from build123d import *

# Parameters (mm, degrees)
SKIZZE1_W                       = 40
SKIZZE1_H                       = 15
SKIZZE1_R                       = 1.75
AUFSATZ_LINEAR_AUSTRAGEN1_DEPTH = 1
FASE1_SIZE                      = 2


with BuildPart() as part:
    # Skizze1 → Aufsatz-Linear austragen1 (new body)
    with BuildSketch(Plane.XY):
        Rectangle(SKIZZE1_W, SKIZZE1_H)
        with Locations((-15, 0)):
            Circle(SKIZZE1_R, mode=Mode.SUBTRACT)
        with Locations((15, 0)):
            Circle(SKIZZE1_R, mode=Mode.SUBTRACT)
    extrude(amount=AUFSATZ_LINEAR_AUSTRAGEN1_DEPTH)

    # Fase1
    fase1_edges = [part.edges().sort_by_distance(p)[0] for p in [
        (-20, 7.5, 0.5),
        (20, 7.5, 0.5),
        (20, -7.5, 0.5),
        (-20, -7.5, 0.5),
    ]]
    chamfer(fase1_edges, length=FASE1_SIZE)


solid = part.part
CAD build for the part. Positions are in the model's coordinates, mm. Round coordinates to 2 decimals unless told otherwise and drop trailing zeros. Order: outer loops, then holes, each group sorted by start corner. A loop starts at its lowest first (then second) coordinate and runs counter-clockwise, first axis right, second up. Notation, with made-up numbers: (6, 38) - (32, 38) arc R24 cw to (32, 70) - close; hole circle Ø10 at (44.25, 38). An arc over 180 degrees is marked (long way). Return JSON: item names as keys, results as strings.
(1) Cut at C-C (y = 0). Give the cut face in (x, z), then the cut area to 3 significant figures.
Answer key:
{"outline": "(-20, 0) - (-16.75, 0) - (-16.75, 1) - (-20, 1) - close; (-13.25, 0) - (13.25, 0) - (13.25, 1) - (-13.25, 1) - close; (16.75, 0) - (20, 0) - (20, 1) - (16.75, 1) - close", "area": "33.0 mm^2"}
(2) Wall check: probe 1 along Y at (x, z) = (-15, 0.5); probe 2 along Y at (x, z) = (-13.5, 0.9); probe 3 along X at (y, z) = (5.75, 0.45). Give the ranges that are in metal, low to high. Write a range as from..to.
Answer key:
{"probe 1": "y = -7.5..-1.75, 1.75..7.5", "probe 2": "y = -7.5..-0.9, 0.9..7.5", "probe 3": "x = -19.75..19.75"}
(3) Pin check, flat tip, straight feed: pin 1 Ø4.5 at (x, y) = (-15, 0) entering from -Z. Stop position of the tip, or through.
Answer key:
{"pin 1": "stops at z = 0"}
(4) Cut at B-B (z = 0.25). Give the cut face in (x, y).
Answer key:
{"outline": "(-20, -5.5) - (-18, -7.5) - (18, -7.5) - (20, -5.5) - (20, 5.5) - (18, 7.5) - (-18, 7.5) - (-20, 5.5) - close; hole circle Ø3.5 at (-15, 0); hole circle Ø3.5 at (15, 0)"}
(5) Pull direction X, two halves, no side cores. Call faces 1 (the face through (-20, -0.1, 0.5)), 2 (the face through (19, -6.5, 0.5)), 3 (the face through (-13.331, 0.526, 0.493)): +X half, -X half, draft (parallel to the pull), parting line (faces both ways), or undercut.
Answer key:
{"face 1": "-X half", "face 2": "+X half", "face 3": "undercut"}
(6) Cut at A-A (x = -15). Give the cut face in (y, z), then the cut area to 3 significant figures.
Answer key:
{"outline": "(-7.5, 0) - (-1.75, 0) - (-1.75, 1) - (-7.5, 1) - close; (1.75, 0) - (7.5, 0) - (7.5, 1) - (1.75, 1) - close", "area": "11.5 mm^2"}
